Geometry: final body of the model. Coordinates: model frame, mm. A direction names the side the tool comes from. Round coordinates to 2 decimals unless told otherwise and drop trailing zeros. Loops run counter-clockwise (first coordinate to the right, second up) from the corner with the lowest first, then second, coordinate; pieces in that order, holes last. Notation, with made-up numbers: M 22.5,-40 L 46.5,-40 A21 ccw 46.5,-23 Z; hole C -6.75,49.25 d3. An arc over 180 degrees is marked long. Write each question's results on one line, items separated by ' | '.
```python
from build123d import *

# Parameters (mm, degrees)
SKETCH1_W               = 25
SKETCH1_H               = 25
SKETCH1_W_2             = 23
SKETCH1_H_2             = 23
BOSS_EXTRUDE1_DEPTH     = 117.5
CUT_EXTRUDE1_DEPTH      = 121.778723292
CUT_EXTRUDE1_DEPTH_BACK = 121.778723292
SKETCH2_R               = 1.5


with BuildPart() as part:
    # Sketch1 → Boss-Extrude1 (new, symmetric)
    with BuildSketch(Plane.XY):
        Rectangle(SKETCH1_W, SKETCH1_H)
        Rectangle(SKETCH1_W_2, SKETCH1_H_2, mode=Mode.SUBTRACT)
    extrude(amount=BOSS_EXTRUDE1_DEPTH, both=True)

    # Sketch2 → Cut-Extrude1 (cut, two sides: drawn at the far end of the back side and taken through both)
    with BuildSketch(Plane(origin=(0, 12.5, 0), x_dir=(1, 0, 0), z_dir=(0, 1, 0)).offset(-CUT_EXTRUDE1_DEPTH_BACK)):
        with Locations(Location((0, 75, 0), (0, 0, 270))):
            Circle(SKETCH2_R)
        with Locations(Location((0, -75, 0), (0, 0, 270))):
            Circle(SKETCH2_R)
    extrude(amount=CUT_EXTRUDE1_DEPTH + CUT_EXTRUDE1_DEPTH_BACK, mode=Mode.SUBTRACT)


solid = part.part
```
1. Section C-C (z = -40). Output: boundary loops of the cut face in (x, y), then the cut area to 3 significant figures.
Answer key:
outline: M -12.5,-12.5 L 12.5,-12.5 L 12.5,12.5 L -12.5,12.5 Z; hole M -11.5,-11.5 L 11.5,-11.5 L 11.5,11.5 L -11.5,11.5 Z | area: 96.0 mm²
2. Section A-A (x = 8.5). Output: boundary loops of the cut face in (y, z).
Answer key:
outline: M -12.5,-117.5 L -11.5,-117.5 L -11.5,117.5 L -12.5,117.5 Z; M 11.5,-117.5 L 12.5,-117.5 L 12.5,117.5 L 11.5,117.5 Z
3. Draft query along Y for faces 1 (the face through (0, -12.5, 2)), 2 (the face through (12.5, 0, 2)), 3 (the face through (-11.5, 0, 2)), 4 (the face through (0, 11.5, 2)). Return one class per face: pulls with the +Y half, pulls with the -Y half, needs draft (parallel to the pull), parting line crosses it, or undercut.
Answer key:
face 1: pulls with the -Y half | face 2: needs draft | face 3: undercut | face 4: undercut
4. Pin query (flat end, axial travel): P1, Ø3.5, axis at x = 0, z = 75, coming from the -Y side. Return the tip coordinate at first contact, or that it passes through.
Answer key:
P1: stops at y = -12.5
5. Access query for faces 5 (the face through (0, -11.5, 2)), 6 (the face through (-1, -12, -117.5)). Directions: +Z, -Z, +X, -X, +Y, -Y. A direction counts if a zero-diameter tool reaches every point of the face in a straight line with its end or side. Return the directions, or none.
Answer key:
face 5: +Z, -Z | face 6: -Z, +X, -X, +Y, -Y
6. Ray query, probe 1 along Z at (x, y) = (0, 12.3); probe 2 along Y at (x, z) = (-8.5, 25); probe 3 along X at (y, z) = (-11.9, 75). Return the intervals inside material, ascending.
Answer key:
probe 1: z = -117.5 to -76.5, -73.5 to 73.5, 76.5 to 117.5 | probe 2: y = -12.5 to -11.5, 11.5 to 12.5 | probe 3: x = -12.5 to -1.5, 1.5 to 12.5
